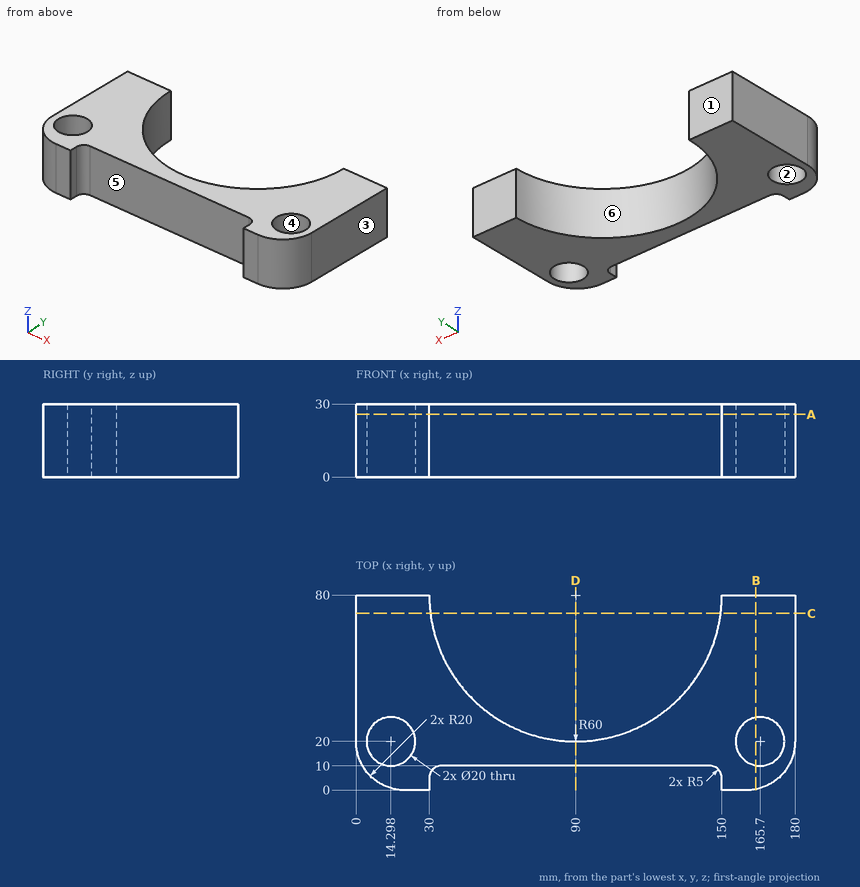
For this review, use the dimensioned drawing (mm, ordinates from the lowest corner) and the shaded views. A direction names the side the tool comes from. Give positions to 0.01 mm unless a question says otherwise; leave off trailing zeros. Order: outer loops, then holes, each group sorted by start corner. A loop starts at its lowest first (then second) coordinate and runs counter-clockwise, first axis right, second up.
1) The part is to be moulded in two halves that separate along Y. For the marked faces 1, 2, 3 and 4, say which applies: released by +Y, released by -Y, zero draft, split by the parting line, or undercut.
2) Wall thickness on line 1 (X direction, y = 26, z = 6.75); line 2 (X direction, y = 63.5, z = 21.5); line 3 (X direction, y = 48.5, z = 5.25): over which ranges is each line inside the solid? List them lowest first.
3) Take a section at C-C (y = 72.5). Give the boundary of the cut face in (x, z), then the cut area to 3 significant figures.
4) Take a section at A-A (z = 25.75). Give the boundary of the cut face in (x, y), then the cut area to 3 significant figures.
5) For the marked faces 5 and 6, list the 3-axis set-ups (+Z, -Z, +X, -X, +Y, -Y) from which the entire face can be reached by the end or side of a thin tool; tool diameter is ignored.
6) Insertion check: pin 1 (16 mm diameter, centred on x = 14.3, y = 20, fed in from +Z); pin 2 (5 mm diameter, centred on x = 156, y = 13, fed in from -Z); pin 3 (1.5 mm diameter, centred on y = 2, z = 11.5, fed in from +X); pin 4 (2.5 mm diameter, centred on y = 2, z = 19, fed in from -X). Each pin has a flat end and moves straight along its axis. Give the tip position at first contact, or say it passes through.
7) Take a section at D-D (x = 90). Give the boundary of the cut face in (y, z), then the cut area to 3 significant figures.
8) Take a section at B-B (x = 164). Give the boundary of the cut face in (y, z), then the cut area to 3 significant figures.
Derived:
1. face 1: released by +Y
1. face 2: undercut
1. face 3: zero draft
1. face 4: undercut
2. line 1: x = 0 to 6.3, 22.3 to 63.85, 116.15 to 157.7, 173.7 to 180
2. line 2: x = 0 to 32.31, 147.69 to 180
2. line 3: x = 0 to 38.93, 141.07 to 180
3. outline: (0, 0) - (30.47, 0) - (30.47, 30) - (0, 30) - close; (149.53, 0) - (180, 0) - (180, 30) - (149.53, 30) - close
3. area: 1,830 mm2
4. outline: (0, 20) arc R20 ccw to (20, 0) - (30, 0) - (30, 5) arc R5 cw to (35, 10) - (145, 10) arc R5 cw to (150, 5) - (150, 0) - (160, 0) arc R20 ccw to (180, 20) - (180, 80) - (150, 80) arc R60 cw to (30, 80) - (0, 80) - close; hole circle Ø20 at (14.3, 20); hole circle Ø20 at (165.7, 20)
4. area: 6,760 mm2
5. face 5: +Z, -Z, -Y
5. face 6: +Z, -Z, +Y
6. pin 1: passes through
6. pin 2: stops at z = 0
6. pin 3: stops at x = 170.12
6. pin 4: stops at x = 9.07
7. outline: (10, 0) - (20, 0) - (20, 30) - (10, 30) - close
7. area: 300 mm2
8. outline: (0.4, 0) - (10.15, 0) - (10.15, 30) - (0.4, 30) - close; (29.85, 0) - (80, 0) - (80, 30) - (29.85, 30) - close
8. area: 1,800 mm2
